Source: three-view drawing plus pictorial views. Frame: mm from the lowest corner of the part. A direction names the side the tool comes from. Round coordinates to 2 decimals unless told otherwise and drop trailing zeros. Order: outer loops, then holes, each group sorted by start corner. A loop starts at its lowest first (then second) coordinate and runs counter-clockwise, first axis right, second up. Notation, with made-up numbers: (6, -14) - (12, -14) arc R11 cw to (12, -5) - close; hole circle Ø8 at (69, 14). An arc over 180 degrees is marked (long way). One line per item, written item: value. Start each with the question number.
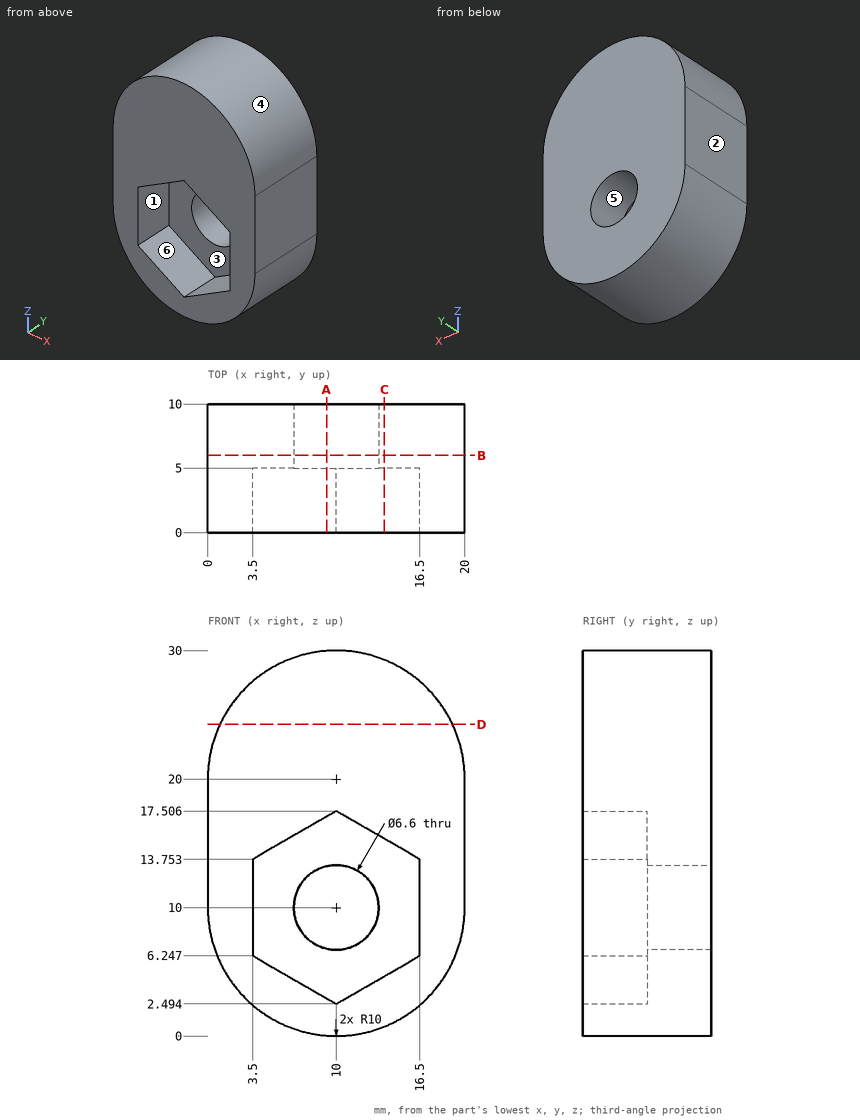
Item 1: Line query: L1, parallel to Z at x = 10, y = 7.9; L2, parallel to X at y = 6.35, z = 10; L3, parallel to Y at x = 9.5, z = 3. Output: solid intervals per line, ascending.
Item 2: Section query D-D on z = 24.25. Return loops of the section in (x, y), and give its area (3 significant figures).
Item 3: Reachability of the marked faces 5 and 6 from +Z, -Z, +X, -X, +Y, -Y: full face, straight path, thin tool, end or side. Return the list, or none.
Item 4: Section query A-A on x = 9.25. Return loops of the section in (y, z).
Item 5: First-contact query: pin 1 Ø3 at (x, y) = (14.5, 4) entering from +Z; pin 2 Ø6 at (y, z) = (2.5, 22) entering from -X; pin 3 Ø10.5 at (x, z) = (10, 10) entering from -Y; pin 4 Ø1.5 at (y, z) = (8.5, 5.5) entering from -X. Flat tips, straight axial feed; report the tip coordinate or a pass-through.
Item 6: Section query B-B on y = 6. Return loops of the section in (x, z).
Item 7: Pull-direction query (Z, two-part tool) for the marked faces 1, 2, 3 and 4; classes: released by +Z, released by -Z, zero draft, split by the parting line, or undercut.
Item 8: Section query C-C on x = 13.75. Return loops of the section in (y, z).
Geometry results:
1. L1: z = 0 to 6.7, 13.3 to 30
1. L2: x = 0 to 6.7, 13.3 to 20
1. L3: y = 5 to 10
2. outline: (0.95, 0) - (19.05, 0) - (19.05, 10) - (0.95, 10) - close
2. area: 181 mm^2
3. face 5: +Y, -Y
3. face 6: -Y
4. outline: (0, 0.03) - (10, 0.03) - (10, 6.79) - (5, 6.79) - (5, 2.93) - (0, 2.93) - close; (0, 17.07) - (5, 17.07) - (5, 13.21) - (10, 13.21) - (10, 29.97) - (0, 29.97) - close
5. pin 1: stops at z = 29.54
5. pin 2: stops at x = 0
5. pin 3: stops at y = 5
5. pin 4: stops at x = 0.73
6. outline: (0, 10) arc R10 ccw to (20, 10) - (20, 20) arc R10 ccw to (0, 20) - close; hole circle Ø6.6 at (10, 10)
7. face 1: undercut
7. face 2: zero draft
7. face 3: undercut
7. face 4: released by +Z
8. outline: (0, 0.73) - (10, 0.73) - (10, 29.27) - (0, 29.27) - (0, 15.34) - (5, 15.34) - (5, 4.66) - (0, 4.66) - close
